CAD build for the part. Positions are in the model's coordinates, mm. A direction names the side the tool comes from. Round coordinates to 2 decimals unless told otherwise and drop trailing zeros. Order: outer loops, then holes, each group sorted by start corner. A loop starts at its lowest first (then second) coordinate and runs counter-clockwise, first axis right, second up. Notation, with made-up numbers: M 45,6.5 L 59,6.5 A24 cw 59,33.5 Z; hole C 31.25,-5 d2. An arc over 180 degrees is marked long. Put each result on its own line as item: value.
Autodesk Inventor part; units mm, degrees
ref_plane "YZ Plane" through (0, 0, 0) normal (1, 0, 0) x (0, 1, 0)
ref_plane "XZ Plane" through (0, 0, 0) normal (0, 1, 0) x (-1, 0, 0)
ref_plane "XY Plane" through (0, 0, 0) normal (0, 0, 1) x (1, 0, 0)
sketch "Sketch1" plane through (0, 0, 0) normal (0, 0, 1) x (1, 0, 0)
  circle A0 centre (0, 0) radius 11.1125
  dimension "d0" = 22.225
extrude "Bearing Offset" add sketch "Sketch1" along normal blind 1.5875
sketch "Sketch2" plane through (0, 0, 1.5875) normal (0, 0, 1) x (1, 0, 0)
  circle A0 centre (0, 0) radius 11.1125
  circle A1 centre (0, 0) radius 11.9063
  dimension "d3" = 23.8125
extrude "Colson Hub (Press Fit)" add sketch "Sketch2" along normal blind 31.75 contours A0 | A1
sketch "Sketch3" plane through (0, 0, 33.3375) normal (0, 0, 1) x (1, 0, 0)
  circle A0 centre (0, 0) radius 11.9063
  circle A1 centre (0, 0) radius 12.7
  dimension "d6" = 25.4
extrude "Colson Retension" add sketch "Sketch3" along normal blind 11.1125 contours A0 | A1
sketch "Sketch4" plane through (0, 0, 0) normal (0, 0, -1) x (-1, 0, 0)
  circle A0 centre (0, 0) radius 11.1125
  line L0 (3.2079, 5.5563) -> (6.4158, 0)
  line L1 (6.4158, 0) -> (3.2079, -5.5563)
  line L2 (3.2079, -5.5563) -> (-3.2079, -5.5563)
  line L3 (-3.2079, -5.5563) -> (-6.4158, 0)
  line L4 (-6.4158, 0) -> (-3.2079, 5.5563)
  line L5 (-3.2079, 5.5563) -> (3.2079, 5.5563)
  dimension "d9" = 11.1125
extrude "7/16\" Hex" cut sketch "Sketch4" against normal through all contours L0 L1 L2 L3 L4 L5
chamfer "End Chamfers" distance 0.7937 angle 45 2 edges at (-11.1125, 0, 0) (-12.7, 0, 44.45)
properties part number "Colson Hub" material "Aluminum 6061"
Item 1: Band-saw the part on A-A on x = 0. Give the cut face in (y, z), and give its area (3 significant figures).
Answers below:
outline: M -12.7,33.34 L -11.91,33.34 L -11.91,1.59 L -11.11,1.59 L -11.11,0.79 L -10.32,0 L -5.56,0 L -5.56,44.45 L -11.91,44.45 L -12.7,43.66 Z; M 5.56,0 L 10.32,0 L 11.11,0.79 L 11.11,1.59 L 11.91,1.59 L 11.91,33.34 L 12.7,33.34 L 12.7,43.66 L 11.91,44.45 L 5.56,44.45 Z
area: 578 mm²
Item 2: Pin check, flat tips, straight feed: P1, Ø10, axis at x = -7.5, z = 31, coming from the +Y side; P2, Ø10, axis at x = -9.5, z = 31, coming from the -Y side; P3, Ø12, axis at x = 9.5, z = 10, coming from the +Y side. Stop position of each tip, or through.
Answers below:
P1: y = 12.32
P2: y = -11.64
P3: y = 11.38
Item 3: Mould opens along Y. For faces 1 (the cylindrical face through (-2.75, 12.4, 38.42)), 2 (the flat face through (0, -5.556, 22)), 3 (the flat face through (5, 3, 44.45)) say: pulls with the +Y half, pulls with the -Y half, needs draft (parallel to the pull), parting line crosses it, or undercut.
Answers below:
face 1: parting line crosses it
face 2: undercut
face 3: needs draft
Item 4: Probe line 1 along Y through (x, z) = (2, 15.5); line 2 along Z through (x, y) = (-11.25, -2.5); line 3 along Y through (x, z) = (3.5, 34). List the from-to ranges inside material, lowest first. Write a range as [from, to].
Answers below:
line 1: [-11.74, -5.56], [5.56, 11.74]
line 2: [1.59, 44.45]
line 3: [-12.21, -5.05], [5.05, 12.21]
Item 5: Band-saw the part on B-B on z = 30.5. Give the cut face in (x, y).
Answers below:
outline: C 0,0 d23.81; hole M -6.42,0 L -3.21,-5.56 L 3.21,-5.56 L 6.42,0 L 3.21,5.56 L -3.21,5.56 Z
Item 6: Tool access for faces 4 (the cylindrical face through (-2.581, 11.623, 17.24)), 5 (the flat face through (4.834, 2.739, 21.914)), 6 (the flat face through (4.4, -4.4, 0)): list every direction of +Z, -Z, +X, -X, +Y, -Y with a clear straight run to the whole face (end or side of a thin tool).
Answers below:
face 4: -Z
face 5: +Z, -Z
face 6: -Z, +X, -X, +Y, -Y
